The model under review builds one solid part; all positions refer to its coordinate system, in mm. A direction names the side the tool comes from. Coordinates: 2 decimals unless noted, no trailing zeros. Write each loop counter-clockwise with the first axis right and the second up, starting at its lowest first coordinate (ties: lowest second). Pieces come first, ordered by that corner, then holes. Notation, with made-up numbers: (68.5, 64) - (79.5, 64) arc R33 ccw to (79.5, 95) - close; hole circle Ø1 at (-11, 41.25). An arc over 180 degrees is marked (long way). Return JSON: item names as keys, results as strings. Group by question number.
(1) We need section C-C on z = 1.4. State the section outline as (x, y) points.
(2) For pin 1 Ø0.9 at (x, z) = (6, 2) entering from +Y; pin 2 Ø0.9 at (y, z) = (-29, 2) entering from +X; pin 3 Ø0.9 at (x, z) = (5.5, 1.5) entering from -Y, all flat-tipped, find the tip position at first contact; note any pin that passes through.
(3) We need section A-A on x = -1.5. State the section outline as (y, z) points, then the cut area to 3 significant figures.
(4) To check wall thickness, follow L1, parallel to Y at x = 5.25, z = 1; L2, parallel to Y at x = -3, z = 0.8; L3, parallel to Y at x = -0.75, z = 1.15. State the ranges of each line that lie inside material, in increasing order. Write a range as from..to.
(5) We need section B-B on y = 7.5. State the section outline as (x, z) points, then the cut area to 3 significant figures.
(6) Tool access review of faces 1 (the face through (6, -27.71, 2)), 2 (the face through (6, 27.71, 2)), 3 (the face through (-6, 2, 2)): name each direction out of +Z, -Z, +X, -X, +Y, -Y from which nothing blocks a thin tool from reaching the whole face with its end or side.
```python
from build123d import *

# Parameters (mm, degrees)
SKETCH1_W               = 15
SKETCH1_H               = 61.42
BOSS_EXTRUDE2_DEPTH     = 3
SKETCH4_W               = 4
SKETCH4_H               = 3
CUT_EXTRUDE2_DEPTH      = 3
MIRROR2_COPY_1_SKETCH_W = 4
MIRROR2_COPY_1_SKETCH_H = 3
MIRROR2_COPY_1_DEPTH    = 3
SKETCH5_W               = 12
SKETCH5_H               = 22.5
CUT_EXTRUDE3_DEPTH      = 3
SKETCH7_R               = 0.9
CUT_EXTRUDE4_DEPTH      = 4


with BuildPart() as part:
    # Sketch1 → Boss-Extrude2 (new body)
    with BuildSketch(Plane.XY):
        Rectangle(SKETCH1_W, SKETCH1_H)
    extrude(amount=BOSS_EXTRUDE2_DEPTH)

    # Sketch4 → Cut-Extrude2 (cut)
    with BuildSketch(Plane.XY.offset(3)):
        with Locations((-5.5, 29.21)):
            Rectangle(SKETCH4_W, SKETCH4_H)
    cut_extrude2 = extrude(amount=-CUT_EXTRUDE2_DEPTH, mode=Mode.SUBTRACT)

    # Mirror1: Cut-Extrude2 across plane
    add(cut_extrude2.mirror(Plane(origin=(0, 0, 0), x_dir=(0, 0, 1), z_dir=(1, 0, 0))), mode=Mode.SUBTRACT)

    # Mirror2: Cut-Extrude2 across plane
    add(cut_extrude2.mirror(Plane.ZX), mode=Mode.SUBTRACT)

    # Mirror2 copy 1 sketch → Mirror2 copy 1 (cut)
    with BuildSketch(Plane(origin=(0, 0, 3), x_dir=(-1, 0, 0), z_dir=(0, 0, 1))):
        with Locations((-5.5, 29.21)):
            Rectangle(MIRROR2_COPY_1_SKETCH_W, MIRROR2_COPY_1_SKETCH_H)
    extrude(amount=-MIRROR2_COPY_1_DEPTH, mode=Mode.SUBTRACT)

    # Sketch5 → Cut-Extrude3 (cut)
    with BuildSketch(Plane.XY.offset(3)):
        with Locations((0, 2.46)):
            Rectangle(SKETCH5_W, SKETCH5_H)
    extrude(amount=-CUT_EXTRUDE3_DEPTH, mode=Mode.SUBTRACT)

    # Sketch7 → Cut-Extrude4 (cut, through all)
    with BuildSketch(Plane(origin=(0, 0, 0), x_dir=(-1, 0, 0), z_dir=(0, 0, -1))):
        with Locations((0.012913573, 16.255029587)):
            Circle(SKETCH7_R)
        with Locations((0.012913573, -10.994970413)):
            Circle(SKETCH7_R)
    extrude(amount=-CUT_EXTRUDE4_DEPTH, mode=Mode.SUBTRACT)


solid = part.part
```
Ans:
{
 "1": {"outline": "(-7.5, -27.71) - (-3.5, -27.71) - (-3.5, -30.71) - (3.5, -30.71) - (3.5, -27.71) - (7.5, -27.71) - (7.5, 27.71) - (3.5, 27.71) - (3.5, 30.71) - (-3.5, 30.71) - (-3.5, 27.71) - (-7.5, 27.71) - close; hole (-6, -8.79) - (6, -8.79) - (6, 13.71) - (-6, 13.71) - close; hole circle Ø1.8 at (-0.01, -10.99); hole circle Ø1.8 at (-0.01, 16.26)"},
 "2": {"pin 1": "y = 27.71", "pin 2": "x = 3.5", "pin 3": "y = -27.71"},
 "3": {"outline": "(-30.71, 0) - (-8.79, 0) - (-8.79, 3) - (-30.71, 3) - close; (13.71, 0) - (30.71, 0) - (30.71, 3) - (13.71, 3) - close", "area": "117 mm²"},
 "4": {"L1": "-27.71..-8.79, 13.71..27.71", "L2": "-30.71..-8.79, 13.71..30.71", "L3": "-30.71..-11.51, -10.48..-8.79, 13.71..15.74, 16.77..30.71"},
 "5": {"outline": "(-7.5, 0) - (-6, 0) - (-6, 3) - (-7.5, 3) - close; (6, 0) - (7.5, 0) - (7.5, 3) - (6, 3) - close", "area": "9.00 mm²"},
 "6": {"face 1": "+Z, -Z, +X, -Y", "face 2": "+Z, -Z, +X, +Y", "face 3": "+Z, -Z"}
}
